```python
from build123d import *

# Parameters (mm, degrees)
SKETCH1_W           = 18
SKETCH1_H           = 18
BOSS_EXTRUDE1_DEPTH = 20
SKETCH2_W           = 8
SKETCH2_H           = 10
CUT_EXTRUDE1_DEPTH  = 13
SKETCH3_W           = 20
SKETCH3_H           = 5
BOSS_EXTRUDE2_DEPTH = 2
LPATTERN1_COUNT     = 6
LPATTERN1_PITCH     = 20
SKETCH4_W           = 20
SKETCH4_H           = 13
BOSS_EXTRUDE3_DEPTH = 2
SKETCH5_W           = 20
SKETCH5_H           = 18
BOSS_EXTRUDE4_DEPTH = 2
SKETCH6_W           = 108
SKETCH6_H           = 2
CUT_EXTRUDE2_DEPTH  = 2
SKETCH7_W           = 122
SKETCH7_H           = 20
BOSS_EXTRUDE5_DEPTH = 6


with BuildPart() as part:
    # Sketch1 → Boss-Extrude1 (new body)
    with BuildSketch(Plane.XY):
        with Locations((9, 9)):
            Rectangle(SKETCH1_W, SKETCH1_H)
    extrude(amount=BOSS_EXTRUDE1_DEPTH)

    # Sketch2 → Cut-Extrude1 (cut)
    with BuildSketch(Plane.XZ):
        with Locations((9, 10)):
            Rectangle(SKETCH2_W, SKETCH2_H)
    extrude(amount=-CUT_EXTRUDE1_DEPTH, mode=Mode.SUBTRACT)

    # Sketch3 → Boss-Extrude2 (add)
    with BuildSketch(Plane(origin=(18, 0, 0), x_dir=(0, 0, -1), z_dir=(1, 0, 0))):
        with Locations((-10, 2.5)):
            Rectangle(SKETCH3_W, SKETCH3_H)
    extrude(amount=BOSS_EXTRUDE2_DEPTH)


with BuildPart() as lpattern1_1:
    # LPattern1: pattern copy
    add(part.part.moved(Location(Vector(1, 0, 0) * (1 * LPATTERN1_PITCH))))


with BuildPart() as lpattern1_2:
    # LPattern1: pattern copy
    add(part.part.moved(Location(Vector(1, 0, 0) * (2 * LPATTERN1_PITCH))))


with BuildPart() as lpattern1_3:
    # LPattern1: pattern copy
    add(part.part.moved(Location(Vector(1, 0, 0) * (3 * LPATTERN1_PITCH))))


with BuildPart() as lpattern1_4:
    # LPattern1: pattern copy
    add(part.part.moved(Location(Vector(1, 0, 0) * (4 * LPATTERN1_PITCH))))


with BuildPart() as lpattern1_5:
    # LPattern1: pattern copy
    add(part.part.moved(Location(Vector(1, 0, 0) * (5 * LPATTERN1_PITCH))))


with BuildPart() as lpattern1_4_1:
    add(lpattern1_4.part)

    # Combine1: union LPattern1_5, part, LPattern1_1, LPattern1_2, LPattern1_3
    add(lpattern1_5.part)
    add(part.part)
    add(lpattern1_1.part)
    add(lpattern1_2.part)
    add(lpattern1_3.part)

    # Sketch4 → Boss-Extrude3 (add)
    with BuildSketch(Plane(origin=(118, 0, 0), x_dir=(0, 0, -1), z_dir=(1, 0, 0))):
        with Locations((-10, 11.5)):
            Rectangle(SKETCH4_W, SKETCH4_H)
    extrude(amount=BOSS_EXTRUDE3_DEPTH)

    # Sketch5 → Boss-Extrude4 (add)
    with BuildSketch(Plane.ZY):
        with Locations((10, 9)):
            Rectangle(SKETCH5_W, SKETCH5_H)
    extrude(amount=BOSS_EXTRUDE4_DEPTH)

    # Sketch6 → Cut-Extrude2 (cut)
    with BuildSketch(Plane(origin=(0, 0, 0), x_dir=(-1, 0, 0), z_dir=(0, -1, 0))):
        with Locations((-59, -10)):
            Rectangle(SKETCH6_W, SKETCH6_H)
    extrude(amount=-CUT_EXTRUDE2_DEPTH, mode=Mode.SUBTRACT)

    # Sketch7 → Boss-Extrude5 (add)
    with BuildSketch(Plane.XZ):
        with Locations((59, 10)):
            Rectangle(SKETCH7_W, SKETCH7_H)
    extrude(amount=BOSS_EXTRUDE5_DEPTH)


solid = lpattern1_4_1.part
```
Model file for the job. Use its own axes, mm. A direction names the side the tool comes from. Coordinates: 2 decimals unless noted, no trailing zeros. Loops run counter-clockwise (first coordinate to the right, second up) from the corner with the lowest first, then second, coordinate; pieces in that order, holes last. Notation, with made-up numbers: (10, 6.25) - (17, 6.25) arc R22 cw to (17, 16.25) - close; hole circle Ø7 at (28, 64.25). An arc over 180 degrees is marked (long way). Answer as a JSON object with one key per item and string values. Group by question number.
(1) Cut at B-B (x = 70.5). Give the cut face in (y, z).
(2) Probe line 1 along X through (y, z) = (13.5, 7); line 2 along Y through (x, z) = (91.5, 6.25); line 3 along Z through (x, y) = (34.5, 0.5). List the from-to ranges inside material, lowest first.
(3) Tool access for faces 4 (the face through (38, 11, 10)), 5 (the face through (93, 6, 10)): list every direction of +Z, -Z, +X, -X, +Y, -Y with a clear straight run to the whole face (end or side of a thin tool).
(4) Two-plate mould, pull along Y, no slides. Class faces 1 (the face through (58, 4, 0)), 2 (the face through (89, 18, 10)), 3 (the face through (33, 6, 10)): released by +Y, released by -Y, zero draft, split by the parting line, or undercut.
(5) Cut at D-D (y = 7.75). State how many separate pieces and enclosed holes the cut face has, then the cut area to 3 significant figures.
(6) Cut at A-A (y = 14.25). Give the cut face in (x, z), then the cut area to 3 significant figures.
(7) Cut at C-C (z = 17.5). Give the cut face in (x, y), then the cut area to 3 significant figures.
Geometry says:
{
 "1": {"outline": "(-6, 0) - (18, 0) - (18, 20) - (-6, 20) - close; hole (0, 5) - (13, 5) - (13, 15) - (0, 15) - close"},
 "2": {"line 1": "x = -2 to 18, 20 to 38, 40 to 58, 60 to 78, 80 to 98, 100 to 120", "line 2": "y = -6 to 0, 13 to 18", "line 3": "z = 0 to 9, 11 to 20"},
 "3": {"face 4": "+Z, -Z, +Y", "face 5": "none"},
 "4": {"face 1": "zero draft", "face 2": "released by +Y", "face 3": "undercut"},
 "5": {"separate pieces": "6", "enclosed holes": "6", "area": "1,760 mm^2"},
 "6": {"outline": "(-2, 0) - (18, 0) - (18, 20) - (-2, 20) - close; (20, 0) - (38, 0) - (38, 20) - (20, 20) - close; (40, 0) - (58, 0) - (58, 20) - (40, 20) - close; (60, 0) - (78, 0) - (78, 20) - (60, 20) - close; (80, 0) - (98, 0) - (98, 20) - (80, 20) - close; (100, 0) - (120, 0) - (120, 20) - (100, 20) - close", "area": "2,240 mm^2"},
 "7": {"outline": "(-2, -6) - (120, -6) - (120, 18) - (100, 18) - (100, 5) - (98, 5) - (98, 18) - (80, 18) - (80, 5) - (78, 5) - (78, 18) - (60, 18) - (60, 5) - (58, 5) - (58, 18) - (40, 18) - (40, 5) - (38, 5) - (38, 18) - (20, 18) - (20, 5) - (18, 5) - (18, 18) - (-2, 18) - close", "area": "2,800 mm^2"}
}
